from build123d import *

# Parameters (mm, degrees)
BOSS_EXTRUDE1_DEPTH = 6
CHAMFER1_SIZE       = 4
CHAMFER1_SIZE2      = 1.865230633


# Read off the part's stored shape, not the designer's step: M5x0.8 Machine Threads Stud1
with BuildPart() as part:
    # Sketch1 → Boss-Extrude1 (new body)
    with BuildSketch(Plane(origin=(0, 0, 0), x_dir=(1, 0, 0), z_dir=(0, 1, 0))):
        Polygon((0, 0), (0, 3.5), (2.1, 3.5), (2.1, 5.3), (8.1, 5.3), (8.1, 3.5), (10.2, 3.5), (10.2, 0), align=None)
    extrude(amount=BOSS_EXTRUDE1_DEPTH)

    # M5x0.8 Machine Threads Stud1 outline → M5x0.8 Machine Threads Stud1 (revolve)
    with BuildSketch(Plane(origin=(5.1, 3, 0), x_dir=(1, 0, 0), z_dir=(0, -1, 0))):
        Polygon((0, -5.3), (0, -15.3), (2.055, -15.3), (2.5, -14.855), (2.5, -5.3), align=None)
    revolve(axis=Axis((5.1, 3, 0), (0, 0, 1)))

    # Chamfer1
    chamfer1_edges = [part.edges().sort_by_distance(p)[0] for p in [
        (0, 3, 0),
        (10.2, 3, 0),
    ]]
    chamfer1_side = [part.faces().sort_by_distance(p)[0] for p in [
        (5.1, 3, 0),
    ]]
    chamfer(chamfer1_edges, length=CHAMFER1_SIZE, length2=CHAMFER1_SIZE2, reference=chamfer1_side[0])


solid = part.part
Input: part model. Units: mm. Frame: model coordinates. A direction names the side the tool comes from. Give positions to 0.01 mm unless a question says otherwise; leave off trailing zeros. Loops run counter-clockwise (first coordinate to the right, second up) from the corner with the lowest first, then second, coordinate; pieces in that order, holes last. Notation, with made-up numbers: (-24, 82) -> (33, 82) arc R12 cw to (33, 87) -> close; hole circle Ø1 at (86.25, 34). An arc over 180 degrees is marked (long way). Answer as a JSON object with one key per item and string values. Group by question number.
Item 1: Cut plane B-B, the plane y = 3. Return the cut outline in (x, z) (3 decimals).
Item 2: Cut plane D-D, the plane x = 8.5. Return the cut outline in (y, z).
Item 3: Pin query (flat end, axial travel): P1, Ø1.7, axis at x = 1.5, y = 3, coming from the -Z side; P2, Ø1, axis at x = 9, y = 2.5, coming from the -Z side; P3, Ø0.5, axis at y = 4.5, z = -4, coming from the +X side. Return the tip coordinate at first contact, or that it passes through.
Item 4: Line query: probe 1 along X at (y, z) = (1.5, -3.75); probe 2 along Y at (x, z) = (5.25, -14); probe 3 along X at (y, z) = (2.9, -9.5). Output: solid intervals per line, ascending.
Item 5: Reachability of faces 1 (the flat face through (2.1, 3, -4)), 2 (the flat face through (8.1, 3, -4)), 3 (the cylindrical face through (3.1, 1.5, -10)) from +Z, -Z, +X, -X, +Y, -Y: full face, straight path, thin tool, end or side. Return the list, or none.
Item 6: Cut plane A-A, the plane x = 5.1. Return the cut outline in (y, z) (3 decimals).
Item 7: Cut plane C-C, the plane z = -11.75. Return the cut outline in (x, y).
Checks:
{
 "1": {"outline": "(0, -3.5) -> (2.1, -3.5) -> (2.1, -5.3) -> (2.6, -5.3) -> (2.6, -14.855) -> (3.045, -15.3) -> (7.155, -15.3) -> (7.6, -14.855) -> (7.6, -5.3) -> (8.1, -5.3) -> (8.1, -3.5) -> (10.2, -3.5) -> (10.2, -1.865) -> (6.2, 0) -> (4, 0) -> (0, -1.865) -> close"},
 "2": {"outline": "(0, -3.5) -> (6, -3.5) -> (6, -1.07) -> (0, -1.07) -> close"},
 "3": {"P1": "stops at z = -5.3", "P2": "stops at z = -3.5", "P3": "stops at x = 8.1"},
 "4": {"probe 1": "x = 2.1 to 8.1", "probe 2": "y = 0.5 to 5.5", "probe 3": "x = 2.6 to 7.6"},
 "5": {"face 1": "-Z, -X, +Y, -Y", "face 2": "-Z, +X, +Y, -Y", "face 3": "-Z"},
 "6": {"outline": "(0, -5.3) -> (0.5, -5.3) -> (0.5, -14.855) -> (0.945, -15.3) -> (5.055, -15.3) -> (5.5, -14.855) -> (5.5, -5.3) -> (6, -5.3) -> (6, 0) -> (0, 0) -> close"},
 "7": {"outline": "circle Ø5 at (5.1, 3)"}
}
